For this review, use the dimensioned drawing (mm, ordinates from the lowest corner) and the shaded views. Round coordinates to 2 decimals unless told otherwise and drop trailing zeros. Loops run counter-clockwise (first coordinate to the right, second up) from the corner with the lowest first, then second, coordinate; pieces in that order, holes last. Notation, with made-up numbers: M -26,89.25 L -1,89.25 A9 ccw -1,106.25 Z; hole C -35,88.25 d11. An arc over 180 degrees is marked long. Answer as a JSON object with one key per item and string values. Group by question number.
Item 1: Consider section B-B (y = 5). State how many separate pieces and enclosed holes the cut face has, and give its area (3 significant figures).
Item 2: Consider section A-A (z = 36). Give the boundary of the cut face in (x, y), and give its area (3 significant figures).
Item 3: To check wall thickness, follow line 1 (Z direction, x = 6, y = 5.5); line 2 (Z direction, x = 42.5, y = 2) (1 decimal); line 3 (X direction, y = 4, z = 92.5). State the ranges of each line that lie inside material, in increasing order.
Item 4: Insertion check: P1, Ø3, axis at x = 41, y = 2, coming from the +Z side (1 decimal); P2, Ø4.5, axis at x = 77.79, z = 96.84, coming from the -Y side. Each pin has a flat end and moves straight along its axis. Give the tip position at first contact, or say it passes through.
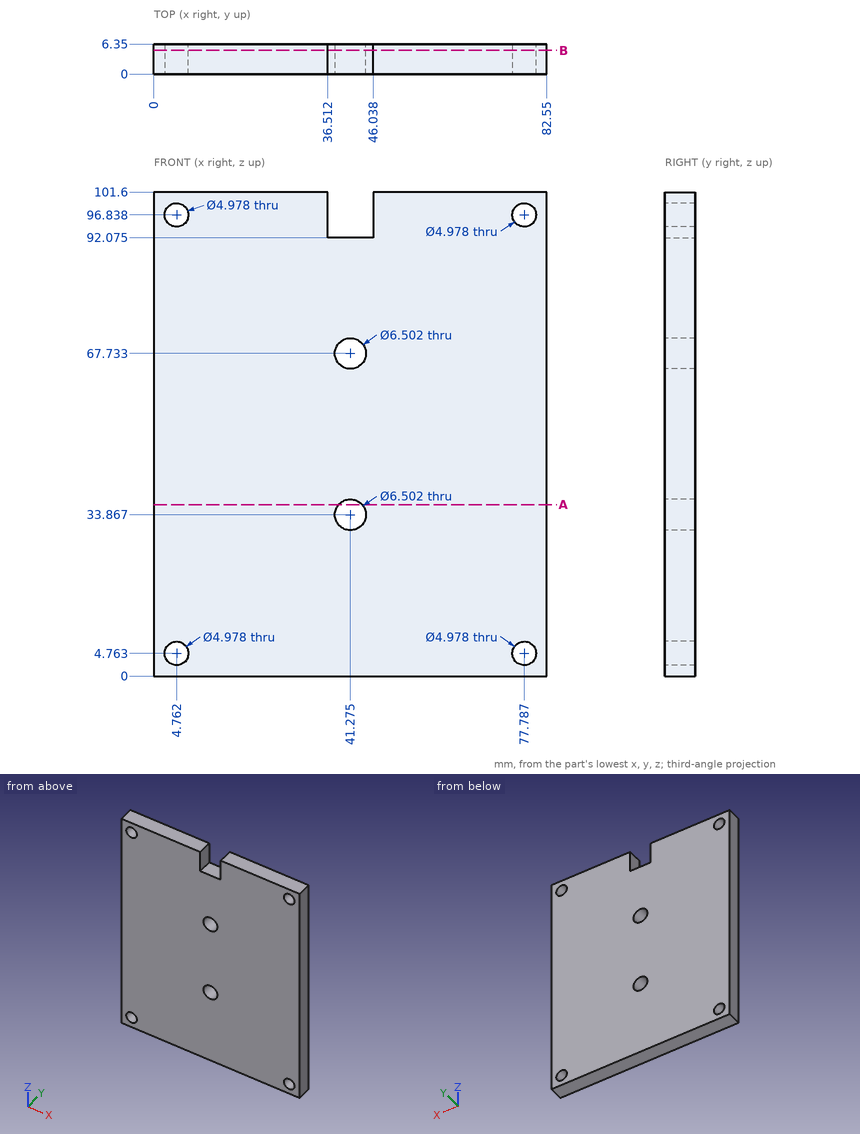
Geometry results:
{
 "1": {"separate pieces": "1", "enclosed holes": "6", "area": "8,150 mm^2"},
 "2": {"outline": "M 0,0 L 38.82,0 L 38.82,6.35 L 0,6.35 Z; M 43.73,0 L 82.55,0 L 82.55,6.35 L 43.73,6.35 Z", "area": "493 mm^2"},
 "3": {"line 1": "z = 0 to 2.6, 6.92 to 94.68, 99 to 101.6", "line 2": "z = 0 to 30.9, 36.9 to 64.7, 70.7 to 92.1", "line 3": "x = 0 to 36.51, 46.04 to 82.55"},
 "4": {"P1": "stops at z = 92.1", "P2": "passes through"}
}
